Here's how the part is built. I have some questions about the finished solid (model axes, mm). Face numbers are marked on the shaded views. A direction names the side the tool comes from. Coordinates: 2 decimals unless noted, no trailing zeros. Write each loop counter-clockwise with the first axis right and the second up, starting at its lowest first coordinate (ties: lowest second). Pieces come first, ordered by that corner, then holes. Notation, with made-up numbers: M -20.5,78.5 L 5.5,78.5 A23 cw 5.5,116.5 Z; hole C 22.25,44 d8. An arc over 180 degrees is marked long. Use a Markdown table: item, result.
```python
from build123d import *

# Parameters (mm, degrees)
SKETCH_1_R                       = 1.49
EXTRUDE_1_DEPTH                  = 4
SKETCH_2_R                       = 2
EXTRUDE_2_DEPTH                  = 4
EXTRUDE_START                    = 4
SKETCH_3_R                       = 2
EXTRUDE_3_DEPTH                  = 4
SKETCH_4_W                       = 4
SKETCH_4_H                       = 2
EXTRUDE_4_DEPTH                  = 12
EXTRUDE_4_DIRECTION_2_REACH      = 10.485
EXTRUDE_4_DIRECTION_2_END_RADIUS = 2
SKETCH_6_W                       = 4
SKETCH_6_H                       = 2
EXTRUDE_5_DEPTH                  = 12
EXTRUDE_5_DIRECTION_2_REACH      = 16.56
EXTRUDE_5_DIRECTION_2_END_RADIUS = 2
CUT_EXTRUDE_1_DEPTH              = 12
CUT_EXTRUDE_1_DEPTH_BACK         = 12
SKETCH_7_W                       = 8
SKETCH_7_H                       = 28
SKETCH_8_R                       = 1
EXTRUDE_6_DEPTH                  = 2


with BuildPart() as part:
    # 草图1 → 凸台-拉伸1 (new body)
    with BuildSketch(Plane.XY):
        Circle(SKETCH_1_R)
    extrude(amount=EXTRUDE_1_DEPTH)

    # 草图2 → 凸台-拉伸2 (add)
    with BuildSketch(Plane(origin=(0, 0, 0), x_dir=(-1, 0, 0), z_dir=(0, 0, -1))):
        Circle(SKETCH_2_R)
    extrude(amount=EXTRUDE_2_DEPTH)

    # 草图3 → 凸台-拉伸3 (add)
    with BuildSketch(Plane.XY.offset(4).offset(EXTRUDE_START)):
        with Locations(Location((0, 0, 0), (0, 0, 180))):
            Circle(SKETCH_3_R)
    extrude(amount=-EXTRUDE_3_DEPTH)

    # 草图4 → 凸台-拉伸4 (add)
    with BuildSketch(Plane(origin=(0, 0, 0), x_dir=(1, 0, 0), z_dir=(0, 1, 0))):
        with Locations((0, 5)):
            Rectangle(SKETCH_4_W, SKETCH_4_H)
    extrude(amount=EXTRUDE_4_DEPTH)

    # 凸台-拉伸4 direction 2: up to this cylinder (the profile starts inside it)
    extrude_4_direction_2_end = Plane(origin=(0, 0, -5), z_dir=(0, 0, 1)) * Cylinder(EXTRUDE_4_DIRECTION_2_END_RADIUS, 25.97, mode=Mode.PRIVATE)
    # 草图4 → 凸台-拉伸4 direction 2 (add, up to the surface)
    with BuildSketch(Plane(origin=(0, 0, 0), x_dir=(1, 0, 0), z_dir=(0, 1, 0)), mode=Mode.PRIVATE) as extrude_4_direction_2_sk1:
        with Locations((0, 5)):
            Rectangle(SKETCH_4_W, SKETCH_4_H)
    extrude_4_direction_2_tool1 = extrude(extrude_4_direction_2_sk1.sketch, amount=-EXTRUDE_4_DIRECTION_2_REACH, mode=Mode.PRIVATE) & extrude_4_direction_2_end
    add(extrude_4_direction_2_tool1.solids().sort_by_distance((0, 0, -5))[0])

    # 草图6 → 凸台-拉伸5 (add)
    with BuildSketch(Plane(origin=(0, 0, 0), x_dir=(1, 0, 0), z_dir=(0, 1, 0))):
        with Locations((0, -9)):
            Rectangle(SKETCH_6_W, SKETCH_6_H)
    extrude(amount=EXTRUDE_5_DEPTH)

    # 凸台-拉伸5 direction 2: up to this cylinder (the profile starts inside it)
    extrude_5_direction_2_end = Plane(origin=(0, 0, 9), z_dir=(0, 0, -1)) * Cylinder(EXTRUDE_5_DIRECTION_2_END_RADIUS, 38.12, mode=Mode.PRIVATE)
    # 草图6 → 凸台-拉伸5 direction 2 (add, up to the surface)
    with BuildSketch(Plane(origin=(0, 0, 0), x_dir=(1, 0, 0), z_dir=(0, 1, 0)), mode=Mode.PRIVATE) as extrude_5_direction_2_sk1:
        with Locations((0, -9)):
            Rectangle(SKETCH_6_W, SKETCH_6_H)
    extrude_5_direction_2_tool1 = extrude(extrude_5_direction_2_sk1.sketch, amount=-EXTRUDE_5_DIRECTION_2_REACH, mode=Mode.PRIVATE) & extrude_5_direction_2_end
    add(extrude_5_direction_2_tool1.solids().sort_by_distance((0, 0, 9))[0])

    # 镜向2: part across plane


with BuildPart() as part_1:
    add(part.part)
    add(part.part.mirror(Plane.ZX.offset(12)))

    # 草图7 → 切除-拉伸1 (cut, two sides: drawn at the far end of the back side and taken through both)
    with BuildSketch(Plane(origin=(0, 0, 0), x_dir=(0, 0, -1), z_dir=(1, 0, 0)).offset(-CUT_EXTRUDE_1_DEPTH_BACK)):
        with Locations((2, 12)):
            Rectangle(SKETCH_7_W, SKETCH_7_H)
    extrude(amount=CUT_EXTRUDE_1_DEPTH + CUT_EXTRUDE_1_DEPTH_BACK, mode=Mode.SUBTRACT)

    # 草图8 → 凸台-拉伸6 (add)
    with BuildSketch(Plane(origin=(0, 0, 2), x_dir=(-1, 0, 0), z_dir=(0, 0, -1))):
        with Locations((0, 24)):
            Circle(SKETCH_8_R)
        Circle(SKETCH_8_R)
    extrude(amount=EXTRUDE_6_DEPTH)


solid = part_1.part
```
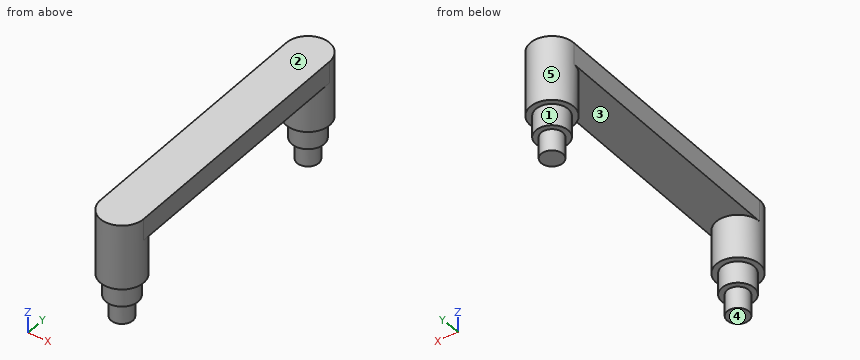
1. Will these pins go through, and if not, where does the flat tip stop? pin 1 Ø2 at (x, y) = (-0.5, 0) entering from -Z; pin 2 Ø1.5 at (x, z) = (1.5, 5.5) entering from -Y; pin 3 Ø1 at (y, z) = (8.5, 6) entering from +X.
Answers follow:
| item | result |
|---|---|
| pin 1 | stops at z = 0 |
| pin 2 | stops at y = -1.85 |
| pin 3 | passes through |
2. I need wall thicknesses on probe 1 along Z at (x, y) = (-1.15, 2.25); probe 2 along Y at (x, z) = (0, 0.75); probe 3 along Y at (x, z) = (-1.25, 5.75). Which ranges of each line are inside material? Lowest first, please.
Answers follow:
| item | result |
|---|---|
| probe 1 | z = 8 to 10 |
| probe 2 | y = -1 to 1, 23 to 25 |
| probe 3 | y = -1.56 to 1.56, 22.44 to 25.56 |
3. Suppose I cut it at A-A on x = 0. Write out the boundary of the cut face in (y, z), and give its area (3 significant figures).
Answers follow:
| item | result |
|---|---|
| outline | M -2,4 L -1.49,4 L -1.49,2 L -1,2 L -1,0 L 1,0 L 1,2 L 1.49,2 L 1.49,4 L 2,4 L 2,8 L 22,8 L 22,4 L 22.51,4 L 22.51,2 L 23,2 L 23,0 L 25,0 L 25,2 L 25.49,2 L 25.49,4 L 26,4 L 26,10 L -2,10 Z |
| area | 108 mm2 |
4. Which directions (+Z, -Z, +X, -X, +Y, -Y) give clear straight access to the entire face, cutting with the end or side of a thin tool? Please do the marked faces 4 and 5.
Answers follow:
| item | result |
|---|---|
| face 4 | -Z, +X, -X, +Y, -Y |
| face 5 | -Z |
5. We'd pull the mould along Y, two halves only. Please class the marked faces 1, 2 and 3: +Y half, -Y half, draft (parallel to the pull), parting line (faces both ways), or undercut.
Answers follow:
| item | result |
|---|---|
| face 1 | undercut |
| face 2 | draft |
| face 3 | undercut |
6. Suppose I cut it at B-B on y = 23.25. Write out the boundary of the cut face in (x, z).
Answers follow:
| item | result |
|---|---|
| outline | M -2,8 L -1.85,8 L -1.85,4 L -1.29,4 L -1.29,2 L -0.66,2 L -0.66,0 L 0.66,0 L 0.66,2 L 1.29,2 L 1.29,4 L 1.85,4 L 1.85,8 L 2,8 L 2,10 L -2,10 Z |
7. Suppose I cut it at C-C on z = 9.75. Write out the boundary of the cut face in (x, y).
Answers follow:
| item | result |
|---|---|
| outline | M -2,0 A2 ccw 2,0 L 2,24 A2 ccw -2,24 Z |
